For this review, take the finished solid that the model builds, in its own axes (mm). Face numbers are marked on the shaded views. Coordinates: 2 decimals unless noted, no trailing zeros. Order: outer loops, then holes, each group sorted by start corner. A loop starts at its lowest first (then second) coordinate and runs counter-clockwise, first axis right, second up. Notation, with made-up numbers: (-7.5, -34.5) - (43.5, -34.5) arc R7 cw to (43.5, -29.5) - close; hole circle Ø9 at (-4.5, -34.75). An arc over 180 degrees is marked (long way). One line per item, written item: value. Start each with the question number.
(1) Consider section D-D on x = -4.5. Write out the cut boundary in (y, z).
(2) Mouldability with a two-part tool opening along X and no side actions: class the marked faces 1, 2, 3 and 4 as released by +X, released by -X, zero draft, split by the parting line, or undercut.
(3) Consider section C-C on x = 4.5. Write out the cut boundary in (y, z), then the cut area to 3 significant figures.
(4) Consider section B-B on z = 3. Write out the cut boundary in (x, y), then the cut area to 3 significant figures.
(5) Consider section A-A on y = 0. Write out the cut boundary in (x, z), then the cut area to 3 significant figures.
(6) To check wall thickness, follow line 1 along Y through (x, z) = (4.5, 3.9); line 2 along Z through (x, y) = (-4.5, 3.75); line 3 along X through (y, z) = (-4.75, 3.35). State the ranges of each line that lie inside material, in increasing order.
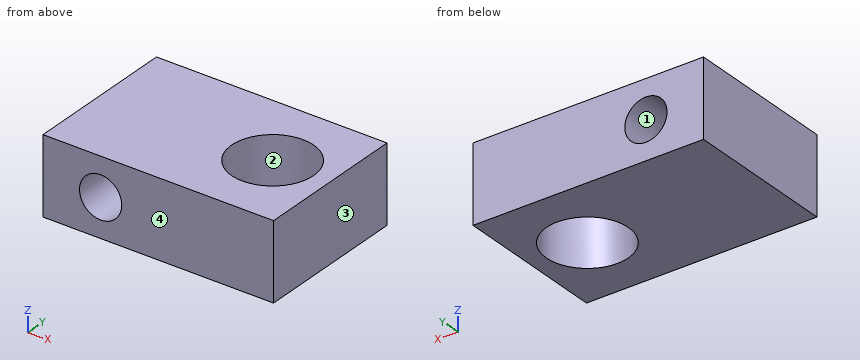
```python
from build123d import *

# Parameters (mm, degrees)
F0_W     = 18
F0_H     = 12
F1_DEPTH = 6
F2_R     = 1.65
F4_DEPTH = 25
F3_R     = 3.2
F5_DEPTH = 25


with BuildPart() as f1:
    # F0 (on Top) → F1 (new body)
    with BuildSketch(Plane.XY):
        Rectangle(F0_W, F0_H)
    extrude(amount=F1_DEPTH)

    # F2 (on face) → F4 (cut)
    with BuildSketch(Plane.XZ.offset(6)):
        with Locations((-4.5, 3)):
            Circle(F2_R)
    extrude(amount=-F4_DEPTH, mode=Mode.SUBTRACT)

    # F3 (on face) → F5 (cut)
    with BuildSketch(Plane.XY.offset(6)):
        with Locations((4.5, 0)):
            Circle(F3_R)
    extrude(amount=-F5_DEPTH, mode=Mode.SUBTRACT)


solid = f1.part
```
Geometry check:
1. outline: (-6, 0) - (6, 0) - (6, 1.35) - (-6, 1.35) - close; (-6, 4.65) - (6, 4.65) - (6, 6) - (-6, 6) - close
2. face 1: undercut
2. face 2: undercut
2. face 3: released by +X
2. face 4: zero draft
3. outline: (-6, 0) - (-3.2, 0) - (-3.2, 6) - (-6, 6) - close; (3.2, 0) - (6, 0) - (6, 6) - (3.2, 6) - close
3. area: 33.6 mm^2
4. outline: (-9, -6) - (-6.15, -6) - (-6.15, 6) - (-9, 6) - close; (-2.85, -6) - (9, -6) - (9, 6) - (-2.85, 6) - close; hole circle Ø6.4 at (4.5, 0)
4. area: 144 mm^2
5. outline: (-9, 0) - (1.3, 0) - (1.3, 6) - (-9, 6) - close; (7.7, 0) - (9, 0) - (9, 6) - (7.7, 6) - close; hole circle Ø3.3 at (-4.5, 3)
5. area: 61.0 mm^2
6. line 1: y = -6 to -3.2, 3.2 to 6
6. line 2: z = 0 to 1.35, 4.65 to 6
6. line 3: x = -9 to -6.11, -2.89 to 9
